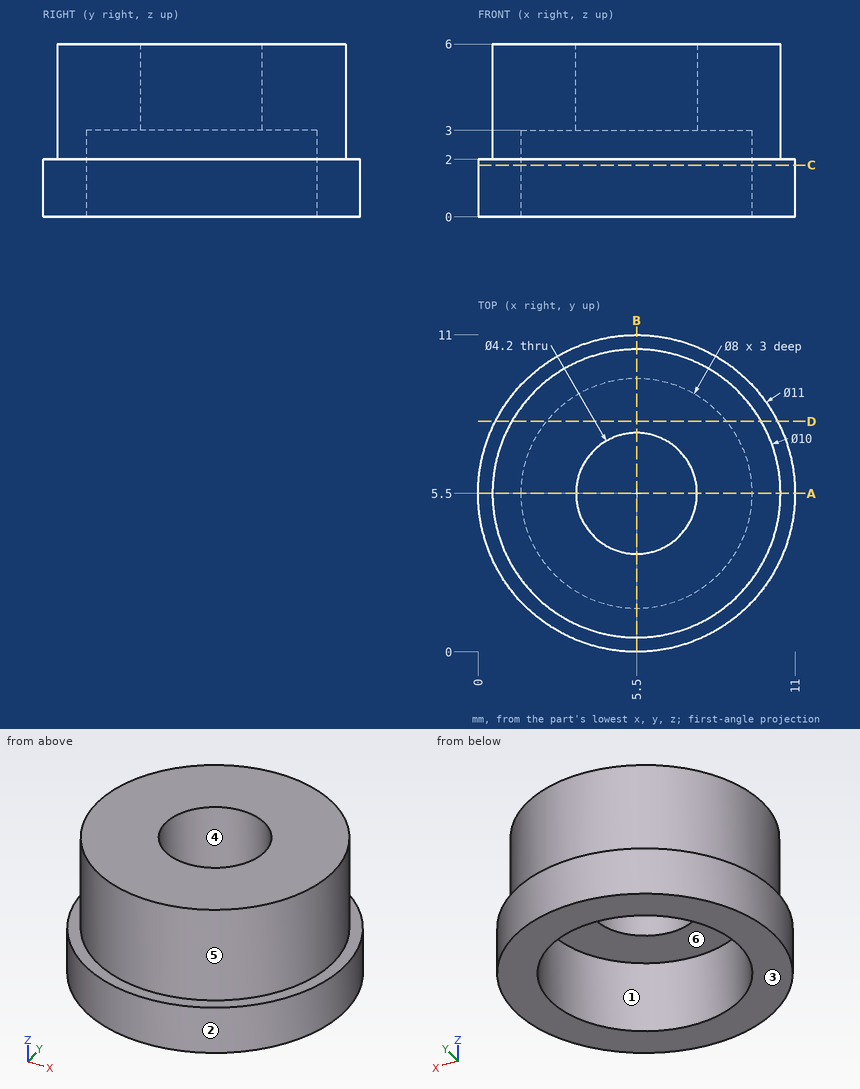
The drawing under review shows one solid part. Ordinate dimensions are in mm from its lowest x, y, z. A direction names the side the tool comes from. Give positions to 0.01 mm unless a question says otherwise; leave off trailing zeros. Order: outer loops, then holes, each group sorted by start corner. A loop starts at its lowest first (then second) coordinate and runs counter-clockwise, first axis right, second up. Notation, with made-up numbers: (85.5, 52) -> (122.5, 52) arc R33 cw to (122.5, 81) -> close; hole circle Ø8 at (-40, 1). An arc over 180 degrees is marked (long way). Write item = value, one per line. Start each with the question number.
(1) To check wall thickness, follow line 1 along Y through (x, z) = (5.5, 1.7); line 2 along Y through (x, z) = (5.5, 4.9); line 3 along Z through (x, y) = (7.25, 3). State the ranges of each line that lie inside material, in increasing order.
(2) For the marked faces 4, 5 and 6, list the 3-axis set-ups (+Z, -Z, +X, -X, +Y, -Y) from which the entire face can be reached by the end or side of a thin tool; tool diameter is ignored.
(3) Mouldability with a two-part tool opening along X and no side actions: class the marked faces 1, 2 and 3 as +X half, -X half, draft (parallel to the pull), parting line (faces both ways), or undercut.
(4) We need section D-D on y = 8. Write out the cut boundary in (x, z).
(5) We need section A-A on y = 5.5. Write out the cut boundary in (x, z).
(6) We need section C-C on z = 1.8. Write out the cut boundary in (x, y), plus the area to 3 significant figures.
(7) For pin 1 (1.5 mm diameter, centred on y = 6, z = 5, fed in from +X); pin 2 (5 mm diameter, centred on x = 5.5, y = 5.5, fed in from -Z), all flat-tipped, find the tip position at first contact; note any pin that passes through.
Numbers:
q1.line_1 = 0 to 1.5, 9.5 to 11
q1.line_2 = 0.5 to 3.4, 7.6 to 10.5
q1.line_3 = 3 to 6
q2.face_4 = +Z, -Z
q2.face_5 = +Z
q2.face_6 = -Z
q3.face_1 = undercut
q3.face_2 = parting line
q3.face_3 = draft
q4.outline = (0.6, 0) -> (2.38, 0) -> (2.38, 3) -> (8.62, 3) -> (8.62, 0) -> (10.4, 0) -> (10.4, 2) -> (9.83, 2) -> (9.83, 6) -> (1.17, 6) -> (1.17, 2) -> (0.6, 2) -> close
q5.outline = (0, 0) -> (1.5, 0) -> (1.5, 3) -> (3.4, 3) -> (3.4, 6) -> (0.5, 6) -> (0.5, 2) -> (0, 2) -> close; (7.6, 3) -> (9.5, 3) -> (9.5, 0) -> (11, 0) -> (11, 2) -> (10.5, 2) -> (10.5, 6) -> (7.6, 6) -> close
q6.outline = circle Ø11 at (5.5, 5.5); hole circle Ø8 at (5.5, 5.5)
q6.area = 44.8 mm^2
q7.pin_1 = 10.5
q7.pin_2 = 3
